Read the model definition and answer for the solid it produces. Units are mm, in the model's axes. Face numbers are marked on the shaded views. A direction names the side the tool comes from. Round coordinates to 2 decimals unless told otherwise and drop trailing zeros. Write each loop counter-clockwise with the first axis right and the second up, starting at its lowest first coordinate (ties: lowest second). Pieces come first, ordered by that corner, then holes.
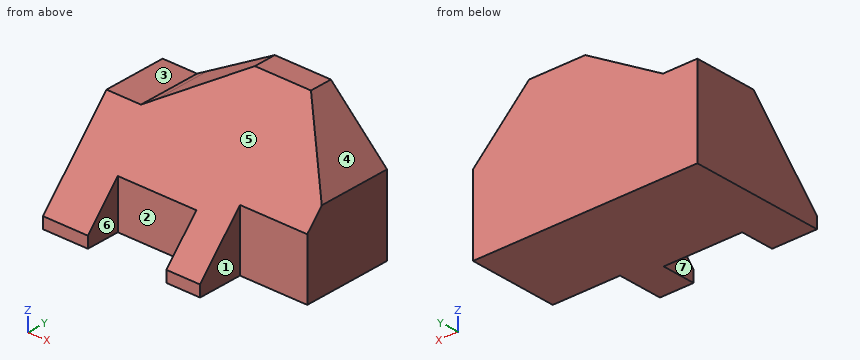
from build123d import *

# Parameters (mm, degrees)
F1_DEPTH = 60
F3_DEPTH = 100.001
F5_DEPTH = 60.001


with BuildPart() as f1:
    # F0 (on Top) → F1 (new body)
    with BuildSketch(Plane.XY):
        Polygon((45, 60), (-55, 60), (-55, 0), (-35, 0), (-35, 15), (0, 15), (0, 0), (15, 0), (15, 20), (45, 20), align=None)
    extrude(amount=-F1_DEPTH)

    # F2 (on face) → F3 (cut, through all)
    with BuildSketch(Plane(origin=(-55, 0, 0), x_dir=(0, -1, 0), z_dir=(-1, 0, 0))):
        Polygon((0, 0), (-50, 0), (0, -55), align=None)
    extrude(amount=-F3_DEPTH, mode=Mode.SUBTRACT)

    # F4 (on Front) → F5 (cut, through all)
    with BuildSketch(Plane.XZ):
        Polygon((-35, 0), (-55, 0), (-55, -20), (-39.641016, -20), (-35, -17.320508), align=None)
        Polygon((-5, 0), (-35, 0), (-35, -17.320508), align=None)
        Polygon((45, -25), (45, 0), (20, 0), align=None)
    extrude(amount=-F5_DEPTH, mode=Mode.SUBTRACT)


solid = f1.part
Q1. Which of the six approach directions +Z, -Z, +X, -X, +Y, -Y give full straight-line access (tool end or side, diameter ignored) to the marked faces 1, 2 and 3?
Verdict:
face 1: +Z, -Z, +X, -Y
face 2: +Z, -Z, -Y
face 3: +Z, -X, +Y, -Y
Q2. Section B-B (x = -43) is taken. Determine the outline of the cut face in (y, z).
Verdict:
outline: (0, -60) - (60, -60) - (60, -20) - (31.82, -20) - (0, -55) - close
Q3. Flat-ended cylindrical pins translate along their axes: pin 1 Ø6 at (x, y) = (30, 51) entering from +Z; pin 2 Ø4.5 at (x, y) = (-46.5, 45.5) entering from +Z; pin 3 Ø5 at (x, z) = (19.5, -16) entering from -Y. Find the tip coordinate at first contact, or state that the pin passes through.
Verdict:
pin 1: stops at z = -7
pin 2: stops at z = -20
pin 3: stops at y = 33.18
Q4. Section C-C (z = -41.5) is taken. Determine the outline of the cut face in (x, y), then the cut area to 3 significant figures.
Verdict:
outline: (-55, 12.27) - (-35, 12.27) - (-35, 15) - (0, 15) - (0, 12.27) - (15, 12.27) - (15, 20) - (45, 20) - (45, 60) - (-55, 60) - close
area: 4,450 mm2
Q5. Straight lines are drawn through the part: probe 1 along Y at (x, z) = (23, -43); probe 2 along Y at (x, z) = (40.5, -25); probe 3 along Z at (x, y) = (-35, 56.5). For each, find the intervals that lie inside material, in ascending order.
Verdict:
probe 1: y = 20 to 60
probe 2: y = 27.27 to 60
probe 3: z = -60 to -17.32
Q6. Determine the mould class of the marked faces 4, 5, 6 and 7 for opening direction X: pulls with the +X half, pulls with the -X half, needs draft (parallel to the pull), parting line crosses it, or undercut.
Verdict:
face 4: pulls with the +X half
face 5: needs draft
face 6: undercut
face 7: undercut
Q7. Section A-A (y = 11) is taken. Determine the outline of the cut face in (x, z).
Verdict:
outline: (-55, -60) - (-35, -60) - (-35, -42.9) - (-55, -42.9) - close; (0, -60) - (15, -60) - (15, -42.9) - (0, -42.9) - close
Q8. Section D-D (y = 42) is taken. Determine the outline of the cut face in (x, z).
Verdict:
outline: (-55, -60) - (45, -60) - (45, -25) - (28.8, -8.8) - (-20.24, -8.8) - (-39.64, -20) - (-55, -20) - close
